The model under review builds one solid part; all positions refer to its coordinate system, in mm. Round coordinates to 2 decimals unless told otherwise and drop trailing zeros. Order: outer loops, then holes, each group sorted by start corner. A loop starts at its lowest first (then second) coordinate and runs counter-clockwise, first axis right, second up.
Autodesk Inventor part; units mm, degrees
ref_plane "Work Plane1" through (0, 30, 0) normal (0, -1, 0) x (1, 0, 0)
ref_plane "YZ Plane" through (0, 0, 0) normal (1, 0, 0) x (0, 1, 0)
ref_plane "XZ Plane" through (0, 0, 0) normal (0, 1, 0) x (-1, 0, 0)
sketch "Sketch2" plane through (0, 0, 0) normal (0, 0, 1) x (1, 0, 0)
  line L0 (0, 0) -> (126, 0)
  line L1 (126, 0) -> (126, 60)
  line L2 (126, 60) -> (0, 60)
  line L3 (0, 60) -> (0, 0)
  dimension "d1" = 126
  dimension "d2" = 60
extrude "Extrusion1" add sketch "Sketch2" along normal blind 7
sketch "Sketch3" plane through (126, 0, 0) normal (1, 0, 0) x (0, 0, -1)
  line L0 (0, 0) -> (-7, 0)
  line L1 (-3.5, 0) -> (-3.5, 11)
  circle A0 centre (-3.5, 11) radius 2
  dimension "d5" = 11
  dimension "d6" = 4
extrude "Extrusion2" cut sketch "Sketch3" against normal blind 5.5
pattern_linear "Rectangular Pattern1" count 2 spacing -120.5 along (1, 0, 0) count 2 spacing 38 along (0, 1, 0) of "Extrusion2"
sketch "Sketch4" plane through (0, 0, 0) normal (0, -1, 0) x (1, 0, 0)
  line L0 (0, 7) -> (126, 7)
  line L1 (0, 0) -> (126, 0)
  line L2 (126, 0) -> (126, 7)
  line L3 (126, 7) -> (0, 7)
  line L4 (0, 7) -> (0, 0)
ref_plane "Work Plane1" through (0, 30, 0) normal (0, -1, 0) x (1, 0, 0)
extrude "Extrusion3" add sketch "Sketch4" along normal blind 1
mirror "Mirror1" about plane through (0, 30, 0) normal (0, -1, 0) of "Extrusion3"
sketch "Sketch5" plane through (0, 0, 0) normal (0, 0, -1) x (-1, 0, 0)
  line L0 (0, 61) -> (-126, 61)
  line L1 (0, -1) -> (0, 61)
  line L2 (0, 30) -> (-63, 30)
  line L3 (-63, 50) -> (-63, 10)
  circle A0 centre (-63, 10) radius 2
  circle A1 centre (-63, 50) radius 2
  point P0 (0, 0)
  dimension "d17" = 40
  dimension "d18" = 4
extrude "Extrusion4" cut sketch "Sketch5" against normal blind 5.5
sketch "Sketch7" plane through (0, 0, 0) normal (0, 0, -1) x (-1, 0, 0)
  line L0 (0, -1) -> (0, 61)
  line L1 (0, 30) -> (-25.15, 30)
  line L2 (0, 30) -> (-5, 30)
  line L3 (-25.15, 30) -> (-20.15, 30)
  line L4 (-12.575, -1) -> (-12.575, 14)
  line L5 (-12.575, -1) -> (2.425, -1) construction
  line L6 (-5.075, 14) -> (-20.15, 14)
  line L7 (-20.15, 14) -> (-20.15, 46)
  line L8 (-20.15, 46) -> (-5.075, 46)
  line L9 (-5.075, 46) -> (-5.075, 14)
  point P0 (0, 0)
  dimension "d29" = 25.15
  dimension "d30" = 5
  dimension "d31" = 5
  dimension "d32" = 15
  dimension "d33" = 90
  dimension "d34" = 32
extrude "Extrusion6" cut sketch "Sketch7" against normal up to surface (7 mm away)
ref_plane "Work Plane2" through (63, -1, 0) normal (-1, 0, 0) x (0, 0, 1)
mirror "Mirror2" about plane through (63, -1, 0) normal (-1, 0, 0) of "Extrusion6"
properties part number "base3"
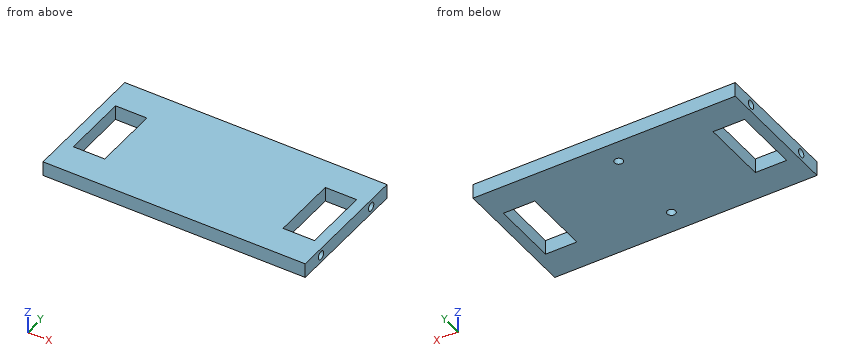
(1) We need section B-B (y = 31). Give the boundary of the cut face in (x, z) (3 decimals), and give its area (3 significant figures).
(2) We need section A-A (z = 3.5). Count the separate pieces of the cut face and the enclosed holes in it, and give its area (3 significant figures).
(3) We need section C-C (x = 117.5). Give the boundary of the cut face in (y, z).
(4) Clearance check with flat-ended pins moving along their axes: P1, Ø3, axis at y = 11, z = 3.5, coming from the -X side; P2, Ø4.5, axis at x = 63, y = 9.5, coming from the -Z side. State where each tip first meets the part, or that it passes through.
(5) To check wall thickness, follow L1, parallel to Y at x = 123.3, z = 3.5; L2, parallel to X at y = 23.5, z = 6.25 (3 decimals); L3, parallel to Y at x = 63, z = 4.45. State the ranges of each line that lie inside material, in increasing order.
(6) We need section D-D (x = 63). Give the boundary of the cut face in (y, z).
Verdict:
1. outline: (0, 0) - (5.075, 0) - (5.075, 7) - (0, 7) - close; (20.15, 0) - (105.85, 0) - (105.85, 7) - (20.15, 7) - close; (120.925, 0) - (126, 0) - (126, 7) - (120.925, 7) - close
1. area: 671 mm2
2. separate pieces: 1
2. enclosed holes: 4
2. area: 6,730 mm2
3. outline: (-1, 0) - (14, 0) - (14, 7) - (-1, 7) - close; (46, 0) - (61, 0) - (61, 7) - (46, 7) - close
4. P1: stops at x = 5.5
4. P2: stops at z = 0
5. L1: y = -1 to 9, 13 to 47, 51 to 61
5. L2: x = 0 to 5.075, 20.15 to 105.85, 120.925 to 126
5. L3: y = -1 to 8, 12 to 48, 52 to 61
6. outline: (-1, 0) - (8, 0) - (8, 5.5) - (12, 5.5) - (12, 0) - (48, 0) - (48, 5.5) - (52, 5.5) - (52, 0) - (61, 0) - (61, 7) - (-1, 7) - close
